Autodesk Inventor part; units mm, degrees
ref_plane "YZ Plane" through (0, 0, 0) normal (1, 0, 0) x (0, 1, 0)
ref_plane "XZ Plane" through (0, 0, 0) normal (0, 1, 0) x (-1, 0, 0)
ref_plane "XY Plane" through (0, 0, 0) normal (0, 0, 1) x (1, 0, 0)
sketch "Sketch2" plane through (0, 0, 0) normal (0, 0, 1) x (1, 0, 0)
  arc A0 (7.4831, 55.3969) -> (-7.4831, 55.3969) centre (0, 55.9) ccw
  circle A1 centre (0, 59.65) radius 1.5
  arc A2 (-44.2335, 34.179) -> (-51.7166, 21.2179) centre (-48.4108, 27.95) ccw
  circle A3 centre (-51.6584, 29.825) radius 1.5
  arc A4 (-51.7166, -21.2179) -> (-44.2335, -34.179) centre (-48.4108, -27.95) ccw
  circle A5 centre (-51.6584, -29.825) radius 1.5
  arc A6 (-7.4831, -55.3969) -> (7.4831, -55.3969) centre (0, -55.9) ccw
  circle A7 centre (0, -59.65) radius 1.5
  arc A8 (44.2335, -34.179) -> (51.7166, -21.2179) centre (48.4108, -27.95) ccw
  circle A9 centre (51.6584, -29.825) radius 1.5
  arc A10 (51.7166, 21.2179) -> (44.2335, 34.179) centre (48.4108, 27.95) ccw
  circle A11 centre (51.6584, 29.825) radius 1.5
  arc A12 (-7.4831, 55.3969) -> (-44.2335, 34.179) centre (0, 0) ccw
  arc A13 (-51.7166, 21.2179) -> (-51.7166, -21.2179) centre (0, 0) ccw
  arc A14 (-44.2335, -34.179) -> (-7.4831, -55.3969) centre (0, 0) ccw
  arc A15 (7.4831, -55.3969) -> (44.2335, -34.179) centre (0, 0) ccw
  arc A16 (51.7166, -21.2179) -> (51.7166, 21.2179) centre (0, 0) ccw
  arc A17 (44.2335, 34.179) -> (7.4831, 55.3969) centre (0, 0) ccw
  dimension "d12" = 3
  dimension "d15" = 360
  dimension "d20" = 55.9
extrude "Extrusion1" add sketch "Sketch2" along normal blind 3
properties part number "base_plate"
Can you work these out from the model? Positions are in its coordinate system, mm. Give positions to 0.01 mm unless a question says otherwise; leave off trailing zeros. Write each loop counter-clockwise with the first axis right and the second up, starting at its lowest first coordinate (ties: lowest second). Pieces come first, ordered by that corner, then holes. Notation, with made-up numbers: (41.5, -38) - (66.5, -38) arc R20 ccw to (66.5, -31) - close; hole circle Ø3 at (43.5, 63.5). An arc over 180 degrees is marked (long way). Write item = value, one per line. Start each with the question number.
1. Imagine slicing it at A-A (x = 0). Please give me the cut outline in (y, z), and give its area (3 significant figures).
2. Imagine slicing it at B-B (y = -59.65). Please give me the cut outline in (x, z), and give its area (3 significant figures).
3. For pin 1 (4 mm diameter, centred on x = 51.66, y = 29.82, fed in from +Z); pin 2 (1 mm diameter, centred on x = -12.5, z = 1, fed in from -Y); pin 3 (1.8 mm diameter, centred on x = -51.66, y = -29.82, fed in from -Z); pin 4 (1.5 mm diameter, centred on x = 25, z = 0.5, fed in from +Y), each with a flat end and sliding along its axis, tell me the tip position at first contact or that it passes through.
4. Thinking about a two-plate mould opening in Y: for faces 1 (the face through (-0.195, 58.163, 1.479)), 2 (the face through (55.9, 0.3, 1.5)), 3 (the face through (-27.69, -48.56, 1.48)), 4 (the face through (27.69, 48.56, 1.48)), which applies, released by +Y, released by -Y, zero draft, split by the parting line, or undercut?
5. Imagine slicing it at C-C (z = 2.3). Count the separate pieces of the cut face and the enclosed holes in it, and give its area (3 significant figures).
6. Please list where these lines run through material, in increasing order: line 1 (Y direction, x = 50.5, z = 2.25); line 2 (Y direction, x = -49, z = 2.25); line 3 (X direction, y = 44, z = 0.5).
7. Imagine slicing it at D-D (x = 48.5). Please give me the cut outline in (y, z).
Worked answers:
q1.outline = (-63.4, 0) - (-61.15, 0) - (-61.15, 3) - (-63.4, 3) - close; (-58.15, 0) - (58.15, 0) - (58.15, 3) - (-58.15, 3) - close; (61.15, 0) - (63.4, 0) - (63.4, 3) - (61.15, 3) - close
q1.area = 362 mm2
q2.outline = (-6.5, 0) - (-1.5, 0) - (-1.5, 3) - (-6.5, 3) - close; (1.5, 0) - (6.5, 0) - (6.5, 3) - (1.5, 3) - close
q2.area = 30.0 mm2
q3.pin_1 = 3
q3.pin_2 = -54.6
q3.pin_3 = through
q3.pin_4 = 50.37
q4.face_1 = undercut
q4.face_2 = undercut
q4.face_3 = released by -Y
q4.face_4 = released by +Y
q5.separate_pieces = 1
q5.enclosed_holes = 6
q5.area = 10,300 mm2
q6.line_1 = -35.15 to -30.78, -28.87 to 28.87, 30.78 to 35.15
q6.line_2 = -35.43 to 35.43
q6.line_3 = -34.48 to 34.48
q7.outline = (-35.45, 0) - (35.45, 0) - (35.45, 3) - (-35.45, 3) - close
